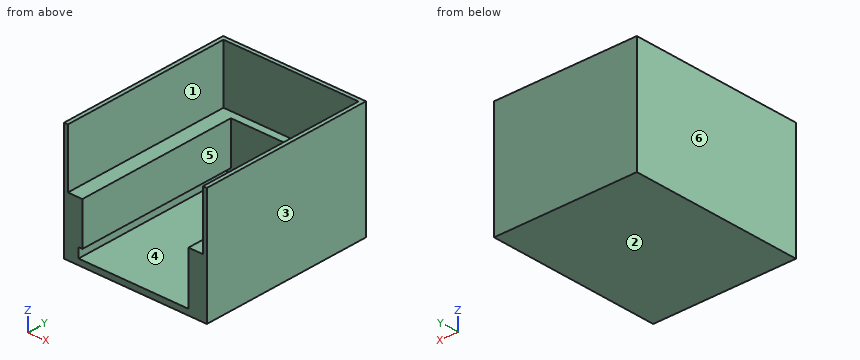
```python
from build123d import *

# Parameters (mm, degrees)
F0_W     = 74
F0_H     = 90
F1_DEPTH = 60
F2_W     = 70
F2_H     = 88
F3_DEPTH = 30
F4_W     = 55
F4_H     = 84
F5_DEPTH = 27
F6_W     = 84
F6_H     = 5
F7_DEPTH = 2


with BuildPart() as f1:
    # F0 (on Top) → F1 (new body)
    with BuildSketch(Plane.XY):
        with Locations((37, -45)):
            Rectangle(F0_W, F0_H)
    extrude(amount=F1_DEPTH)

    # F2 (on face) → F3 (cut)
    with BuildSketch(Plane.XY.offset(60)):
        with Locations((37, -46)):
            Rectangle(F2_W, F2_H)
    extrude(amount=-F3_DEPTH, mode=Mode.SUBTRACT)

    # F4 (on face) → F5 (cut)
    with BuildSketch(Plane.XY.offset(30)):
        with Locations((37, -48)):
            Rectangle(F4_W, F4_H)
    extrude(amount=-F5_DEPTH, mode=Mode.SUBTRACT)

    # F6 (on face) → F7 (cut)
    with BuildSketch(Plane.YZ.offset(9.5)):
        with Locations((-48, 5.5)):
            Rectangle(F6_W, F6_H)
    extrude(amount=-F7_DEPTH, mode=Mode.SUBTRACT)


solid = f1.part
```
Read the model definition and answer for the solid it produces. Units are mm, in the model's axes. Face numbers are marked on the shaded views. A direction names the side the tool comes from. Round coordinates to 2 decimals unless told otherwise and drop trailing zeros. Loops run counter-clockwise (first coordinate to the right, second up) from the corner with the lowest first, then second, coordinate; pieces in that order, holes last. Notation, with made-up numbers: (26, 76.5) -> (73, 76.5) arc R9 ccw to (73, 91.5) -> close; hole circle Ø11 at (64, 32.5). An arc over 180 degrees is marked (long way). One line per item, written item: value.
1) A cutting plane is placed at C-C (y = -42). Determine the outline of the cut face in (x, z), and give its area (3 significant figures).
Answer list:
outline: (0, 0) -> (74, 0) -> (74, 60) -> (72, 60) -> (72, 30) -> (64.5, 30) -> (64.5, 3) -> (7.5, 3) -> (7.5, 8) -> (9.5, 8) -> (9.5, 30) -> (2, 30) -> (2, 60) -> (0, 60) -> close
area: 845 mm²
2) A cutting plane is placed at A-A (x = 17). Determine the outline of the cut face in (y, z), and give its area (3 significant figures).
Answer list:
outline: (-90, 0) -> (0, 0) -> (0, 60) -> (-2, 60) -> (-2, 30) -> (-6, 30) -> (-6, 3) -> (-90, 3) -> close
area: 492 mm²
3) A cutting plane is placed at B-B (z = 5.5). Determine the outline of the cut face in (x, y), and give its area (3 significant figures).
Answer list:
outline: (0, -90) -> (7.5, -90) -> (7.5, -6) -> (64.5, -6) -> (64.5, -90) -> (74, -90) -> (74, 0) -> (0, 0) -> close
area: 1,870 mm²
4) Flat-ended cylindrical pins translate along their axes: P1, Ø10, axis at x = 53.5, z = 33, coming from the -Y side; P2, Ø17, axis at x = 22.5, y = -56.5, coming from the +Z side; P3, Ø24, axis at x = 42, z = 49, coming from the -Y side. Find the tip coordinate at first contact, or state that the pin passes through.
Answer list:
P1: stops at y = -6
P2: stops at z = 3
P3: stops at y = -2
5) For the marked faces 5 and 6, determine the directions among +Z, -Z, +X, -X, +Y, -Y from which every point of the face is accessible in a straight line to the end or side of a thin tool.
Answer list:
face 5: +Z, -Y
face 6: +Z, -Z, -X, +Y, -Y
6) The mould has two halves that part along X. Classify the marked faces 1, 2, 3 and 4: pulls with the +X half, pulls with the -X half, needs draft (parallel to the pull), parting line crosses it, or undercut.
Answer list:
face 1: undercut
face 2: needs draft
face 3: pulls with the +X half
face 4: undercut
7) Consider L1, parallel to X at y = -84, z = 22.5; L2, parallel to X at y = -66.5, z = 34; L3, parallel to Y at x = 14, z = 49. Determine where each line is inside the solid, lowest interval first. Write a range as [from, to].
Answer list:
L1: x = [0, 9.5], [64.5, 74]
L2: x = [0, 2], [72, 74]
L3: y = [-2, 0]
